Source: CAD feature listing. Evaluate the final solid. Frame: model axes, mm. Face numbers are marked on the shaded views. A direction names the side the tool comes from. Give positions to 0.01 mm unless a question says otherwise; leave off trailing zeros. Order: outer loops, then holes, each group sorted by start corner. A loop starts at its lowest first (then second) coordinate and runs counter-clockwise, first axis right, second up. Notation, with made-up numbers: M -14.5,58.25 L -4.5,58.25 A14 cw -4.5,69.25 Z; hole C -25,80 d9. An arc over 180 degrees is marked long. Use CSV: the item, a comma, the result in double quotes. Start each with the question number.
1. Section query A-A, the plane z = -7.5. Return the cut outline in (x, y), plus the area to 3 significant figures.
2. Section query B-B, the plane y = 3.5. Return the cut outline in (x, z), plus the area to 3 significant figures.
3. Pin query (flat end, axial travel): P1, Ø16, axis at x = 37, y = 20.5, coming from the +Z side; P2, Ø6, axis at x = 33, y = 16.5, coming from the -Z side; P3, Ø2.5, axis at x = 45.5, y = 2.5, coming from the -Z side. Return the tip coordinate at first contact, or that it passes through.
4. Section query C-C, the plane x = 26.5. Return the cut outline in (y, z).
5. Section query D-D, the plane z = -20. Return the cut outline in (x, y).
6. Line query: line 1 along X through (y, z) = (5.25, -7.5); line 2 along Y through (x, z) = (25.5, -27); line 3 along X through (y, z) = (17.5, -21). Output: solid intervals per line, ascending. Write a range as [from, to].
7. Mould query, pull axis Y, two halves, no side actions, for the marked faces 1, 2 and 3. Classes: released by +Y, released by -Y, zero draft, split by the parting line, or undercut.
8. Reachability of the marked faces 4, 5, 6, 7 and 8 from +Z, -Z, +X, -X, +Y, -Y: full face, straight path, thin tool, end or side. Return the list, or none.
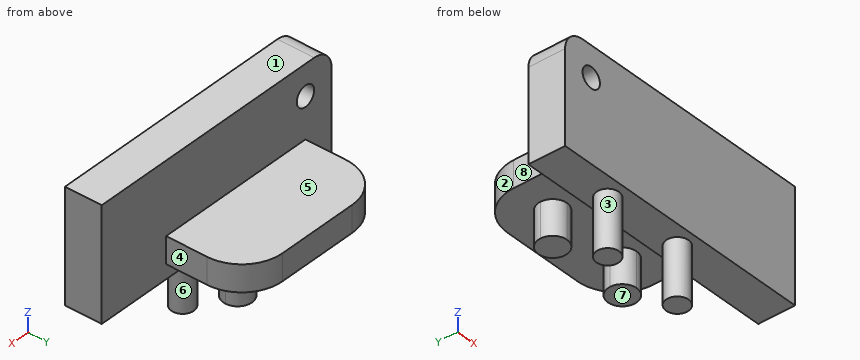
from build123d import *

# Parameters (mm, degrees)
BOSS_EXTRUDE2_DEPTH      = 8
BOSS_EXTRUDE2_DEPTH_BACK = 1
SKETCH1_R                = 2.5
CUT_EXTRUDE1_START       = -16
SKETCH2_R                = 2.5
CUT_EXTRUDE1_DEPTH       = 16
SKETCH3_R                = 2.75
BOSS_EXTRUDE3_DEPTH      = 13.75
SKETCH4_W                = 4.5
SKETCH4_H                = 6.5
BOSS_EXTRUDE4_DEPTH      = 15
BOSS_EXTRUDE5_DEPTH      = 8.5
SKETCH8_W                = 9
SKETCH8_H                = 6.5
BOSS_EXTRUDE6_DEPTH      = 5
SKETCH9_W                = 15.5
SKETCH9_H                = 6.5
BOSS_EXTRUDE7_DEPTH      = 20
BOSS_EXTRUDE8_DEPTH      = 8.5
CUT_EXTRUDE2_START       = -8.5
SKETCH12_R               = 3.5
CUT_EXTRUDE2_DEPTH       = 8.5
FILLET1_R                = 10
BOSS_EXTRUDE9_DEPTH      = 11
BOSS_EXTRUDE9_DEPTH_BACK = 11
SKETCH13_W               = 27.5
SKETCH13_H               = 9


with BuildPart() as part:
    # Sketch1 → Boss-Extrude2 (new, two sides: drawn at the far end of the back side and taken through both)
    with BuildSketch(Plane(origin=(0, 0, 0), x_dir=(1, 0, 0), z_dir=(0, 1, 0)).offset(-BOSS_EXTRUDE2_DEPTH_BACK)):
        with BuildLine():
            Line((5, 0), (50, 0))
            ThreePointArc((50, 0), (53.535533906, 1.464466094), (55, 5))
            Line((55, 5), (55, 50))
            ThreePointArc((55, 50), (53.535533906, 53.535533906), (50, 55))
            Line((50, 55), (5, 55))
            ThreePointArc((5, 55), (1.464466094, 53.535533906), (0, 50))
            Line((0, 50), (0, 5))
            ThreePointArc((0, 5), (1.464466094, 1.464466094), (5, 0))
        make_face()
        with Locations(Location((7.5, 47.5, 0), (0, 0, 270))):
            Circle(SKETCH1_R, mode=Mode.SUBTRACT)
        with Locations(Location((47.5, 47.5, 0), (0, 0, 270))):
            Circle(SKETCH1_R, mode=Mode.SUBTRACT)
        with Locations(Location((47.5, 7.5, 0), (0, 0, 270))):
            Circle(SKETCH1_R, mode=Mode.SUBTRACT)
        with Locations(Location((7.5, 7.5, 0), (0, 0, 270))):
            Circle(SKETCH1_R, mode=Mode.SUBTRACT)
    extrude(amount=BOSS_EXTRUDE2_DEPTH + BOSS_EXTRUDE2_DEPTH_BACK)

    # Sketch2 → Cut-Extrude1 (cut)
    with BuildSketch(Plane(origin=(0, 8, 0), x_dir=(1, 0, 0), z_dir=(0, 1, 0)).offset(CUT_EXTRUDE1_START)):
        with BuildLine():
            Line((0, 50), (0, 27.5))
            Line((0, 27.5), (55, 27.5))
            Line((55, 27.5), (55, 50))
            ThreePointArc((55, 50), (53.535533906, 53.535533906), (50, 55))
            Line((50, 55), (5, 55))
            ThreePointArc((5, 55), (1.464466094, 53.535533906), (0, 50))
        make_face()
        with Locations((7.5, 47.5)):
            Circle(SKETCH2_R, mode=Mode.SUBTRACT)
        with Locations((47.5, 47.5)):
            Circle(SKETCH2_R, mode=Mode.SUBTRACT)
    extrude(amount=CUT_EXTRUDE1_DEPTH, mode=Mode.SUBTRACT)

    # Sketch3 → Boss-Extrude3 (add)
    with BuildSketch(Plane(origin=(0, 0, -27.5), x_dir=(-1, 0, 0), z_dir=(0, 0, -1))):
        with Locations(Location((-37.5, 3.5, 0), (0, 0, 180))):
            Circle(SKETCH3_R)
        with Locations(Location((-17.5, 3.5, 0), (0, 0, 180))):
            Circle(SKETCH3_R)
    extrude(amount=BOSS_EXTRUDE3_DEPTH)

    # Sketch4 → Boss-Extrude4 (add)
    with BuildSketch(Plane(origin=(0, 8, 0), x_dir=(1, 0, 0), z_dir=(0, 1, 0))):
        with Locations((25.25, 20.75)):
            Rectangle(SKETCH4_W, SKETCH4_H)
        with Locations((29.75, 20.75)):
            Rectangle(SKETCH4_W, SKETCH4_H)
    extrude(amount=BOSS_EXTRUDE4_DEPTH)

    # Sketch5 → Boss-Extrude5 (add)
    with BuildSketch(Plane(origin=(0, 0, -24), x_dir=(-1, 0, 0), z_dir=(0, 0, -1))):
        with BuildLine():
            ThreePointArc((-25.636419782, 13.037388184), (-24.436298745, 14.307742745), (-24, 16))
            ThreePointArc((-24, 16), (-29.974873734, 18.474873734), (-27.5, 12.5))
            ThreePointArc((-27.5, 12.5), (-26.685966178, 12.595980474), (-25.916578842, 12.878657751))
            ThreePointArc((-25.916578842, 12.878657751), (-25.85405917, 13.094916041), (-25.636419782, 13.037388184))
        make_face()
    extrude(amount=BOSS_EXTRUDE5_DEPTH)

    # Sketch8 → Boss-Extrude6 (add)
    with BuildSketch(Plane(origin=(0, 23, 0), x_dir=(1, 0, 0), z_dir=(0, 1, 0))):
        with Locations((27.5, 20.75)):
            Rectangle(SKETCH8_W, SKETCH8_H)
    extrude(amount=BOSS_EXTRUDE6_DEPTH)

    # Sketch9 → Boss-Extrude7 (add)
    with BuildSketch(Plane(origin=(0, 8, 0), x_dir=(1, 0, 0), z_dir=(0, 1, 0))):
        with Locations((15.25, 20.75)):
            Rectangle(SKETCH9_W, SKETCH9_H)
        with Locations((39.75, 20.75)):
            Rectangle(SKETCH9_W, SKETCH9_H)
    extrude(amount=BOSS_EXTRUDE7_DEPTH)

    # Sketch10 → Boss-Extrude8 (add)
    with BuildSketch(Plane(origin=(0, 0, -24), x_dir=(-1, 0, 0), z_dir=(0, 0, -1))):
        with BuildLine():
            Line((-21, 17), (-17.5, 17))
            Line((-17.5, 17), (-14, 17))
            ThreePointArc((-14, 17), (-17.5, 20.5), (-21, 17))
        make_face()
        with BuildLine():
            Line((-17.5, 13.5), (-17.5, 17))
            Line((-17.5, 17), (-21, 17))
            ThreePointArc((-21, 17), (-19.974873734, 14.525126266), (-17.5, 13.5))
        make_face()
        with BuildLine():
            Line((-14, 17), (-17.5, 17))
            Line((-17.5, 17), (-17.5, 13.5))
            ThreePointArc((-17.5, 13.5), (-15.025126266, 14.525126266), (-14, 17))
        make_face()
        with BuildLine():
            Line((-37.5, 17), (-34, 17))
            ThreePointArc((-34, 17), (-37.5, 20.5), (-41, 17))
            Line((-41, 17), (-37.5, 17))
        make_face()
        with BuildLine():
            ThreePointArc((-37.5, 13.5), (-35.025126266, 14.525126266), (-34, 17))
            Line((-34, 17), (-37.5, 17))
            Line((-37.5, 17), (-37.5, 13.5))
        make_face()
        with BuildLine():
            Line((-37.5, 13.5), (-37.5, 17))
            Line((-37.5, 17), (-41, 17))
            ThreePointArc((-41, 17), (-39.974873734, 14.525126266), (-37.5, 13.5))
        make_face()
    extrude(amount=BOSS_EXTRUDE8_DEPTH)

    # Sketch12 → Cut-Extrude2 (cut)
    with BuildSketch(Plane(origin=(0, 0, -32.5), x_dir=(-1, 0, 0), z_dir=(0, 0, -1)).offset(CUT_EXTRUDE2_START)):
        with Locations((-27.5, 16)):
            Circle(SKETCH12_R)
    extrude(amount=CUT_EXTRUDE2_DEPTH, mode=Mode.SUBTRACT)

    # Fillet1
    fillet1_edges = [part.edges().sort_by_distance(p)[0] for p in [
        (7.5, 28, -20.75),
        (47.5, 28, -20.75),
    ]]
    fillet(fillet1_edges, radius=FILLET1_R)

    # Sketch13 → Boss-Extrude9 (add, two sides: drawn at the far end of the back side and taken through both)
    with BuildSketch(Plane(origin=(55, 0, 0), x_dir=(0, 0, -1), z_dir=(1, 0, 0)).offset(-BOSS_EXTRUDE9_DEPTH_BACK)):
        with Locations((13.75, 3.5)):
            Rectangle(SKETCH13_W, SKETCH13_H)
    extrude(amount=BOSS_EXTRUDE9_DEPTH + BOSS_EXTRUDE9_DEPTH_BACK)


solid = part.part
Result set:
1,outline,"M 0,-1 L 5,-1 L 5,8 L 0,8 Z; M 10,-1 L 66,-1 L 66,8 L 10,8 Z"
1,area,"549 mm2"
2,outline,"M 0,-27.5 L 14.75,-27.5 L 14.75,-41.25 L 20.25,-41.25 L 20.25,-27.5 L 34.75,-27.5 L 34.75,-41.25 L 40.25,-41.25 L 40.25,-27.5 L 66,-27.5 L 66,0 L 5,0 A5 ccw 0,-5 Z; hole C 7.5,-7.5 d5"
2,area,"1,940 mm2"
3,P1,"z = -17.5"
3,P2,"z = -32.5"
3,P3,"z = -27.5"
4,outline,"M -1,-27.5 L 8,-27.5 L 8,-24 L 28,-24 L 28,-17.5 L 8,-17.5 L 8,0 L -1,0 Z"
5,outline,"M 0,-1 L 66,-1 L 66,8 L 47.5,8 L 47.5,18 A10 ccw 37.5,28 L 17.5,28 A10 ccw 7.5,18 L 7.5,8 L 0,8 Z"
6,line 1,"[0, 5], [10, 66]"
6,line 2,"[-1, 8]"
6,line 3,"[7.5, 47.5]"
7,face 1,"zero draft"
7,face 2,"released by +Y"
7,face 3,"undercut"
8,face 4,"+Z, -Z, +X, +Y"
8,face 5,"+Z, +X, -X, +Y"
8,face 6,"-Z"
8,face 7,"-Z, +X, -X, +Y"
8,face 8,"+Z, -Z, -X, +Y"
